Source: CAD feature listing. Evaluate the final solid. Frame: model axes, mm. Coordinates: 2 decimals unless noted, no trailing zeros. Order: outer loops, then holes, each group sorted by start corner. A loop starts at its lowest first (then second) coordinate and runs counter-clockwise, first axis right, second up.
```python
from build123d import *

# Parameters (mm, degrees)
SKETCH1_W           = 20
SKETCH1_H           = 20
BOSS_EXTRUDE1_DEPTH = 116
SKETCH1_5_R         = 1
CUT_EXTRUDE1_DEPTH  = 10
SKETCH4_R           = 1
CUT_EXTRUDE2_DEPTH  = 10
SKETCH5_R           = 2.5
CUT_EXTRUDE3_DEPTH  = 21
SKETCH6_R           = 5
CUT_EXTRUDE4_DEPTH  = 10


with BuildPart() as part:
    # Sketch1 → Boss-Extrude1 (new body)
    with BuildSketch(Plane.XY):
        with Locations((10, 10)):
            Rectangle(SKETCH1_W, SKETCH1_H)
    extrude(amount=BOSS_EXTRUDE1_DEPTH)

    # Sketch1_5 → Cut-Extrude1 (cut)
    with BuildSketch(Plane.XY):
        with Locations((15, 10)):
            Circle(SKETCH1_5_R)
        with Locations((5, 10)):
            Circle(SKETCH1_5_R)
    extrude(amount=CUT_EXTRUDE1_DEPTH, mode=Mode.SUBTRACT)

    # Sketch4 → Cut-Extrude2 (cut)
    with BuildSketch(Plane.XY.offset(116)):
        with Locations((5, 10)):
            Circle(SKETCH4_R)
        with Locations((15, 10)):
            Circle(SKETCH4_R)
    extrude(amount=-CUT_EXTRUDE2_DEPTH, mode=Mode.SUBTRACT)

    # Sketch5 → Cut-Extrude3 (cut, through all)
    with BuildSketch(Plane(origin=(20, 0, 0), x_dir=(0, 0, -1), z_dir=(1, 0, 0))):
        with Locations((-98, 10)):
            Circle(SKETCH5_R)
        with Locations((-18, 10)):
            Circle(SKETCH5_R)
    extrude(amount=-CUT_EXTRUDE3_DEPTH, mode=Mode.SUBTRACT)

    # Sketch6 → Cut-Extrude4 (cut)
    with BuildSketch(Plane(origin=(20, 0, 0), x_dir=(0, 0, -1), z_dir=(1, 0, 0))):
        with Locations((-98, 10)):
            Circle(SKETCH6_R)
        with Locations((-18, 10)):
            Circle(SKETCH6_R)
    extrude(amount=-CUT_EXTRUDE4_DEPTH, mode=Mode.SUBTRACT)


solid = part.part
```
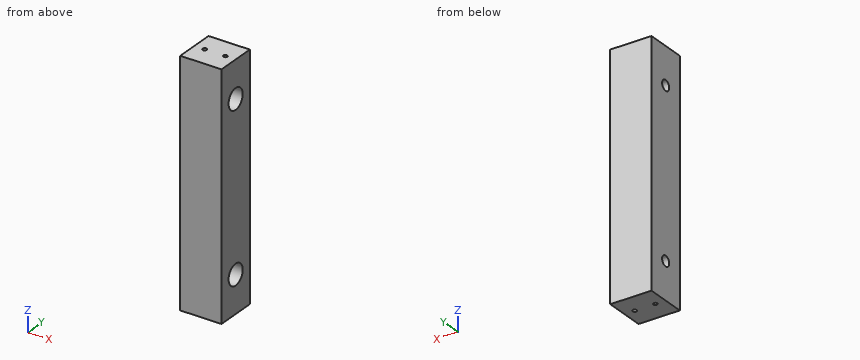
Q1. Pin query (flat end, axial travel): P1, Ø5, axis at y = 11, z = 16, coming from the +X side; P2, Ø1.8, axis at x = 15, y = 10, coming from the +Z side; P3, Ø12, axis at x = 12, y = 12.5, coming from the -Z side; P4, Ø1.6, axis at x = 5, y = 10, coming from the -Z side. Return the tip coordinate at first contact, or that it passes through.
Solutions:
P1: stops at x = 10
P2: stops at z = 106
P3: stops at z = 0
P4: stops at z = 10
Q2. Section query D-D on x = 5. Output: boundary loops of the cut face in (y, z).
Solutions:
outline: (0, 0) - (9, 0) - (9, 10) - (11, 10) - (11, 0) - (20, 0) - (20, 116) - (11, 116) - (11, 106) - (9, 106) - (9, 116) - (0, 116) - close; hole circle Ø5 at (10, 18); hole circle Ø5 at (10, 98)
Q3. Section query C-C on y = 10. Give the number of separate pieces and of enclosed holes in the cut face, plus the area to 3 significant figures.
Solutions:
separate pieces: 3
enclosed holes: 0
area: 1,940 mm2
Q4. Section query B-B on x = 15. Output: boundary loops of the cut face in (y, z).
Solutions:
outline: (0, 0) - (9, 0) - (9, 10) - (11, 10) - (11, 0) - (20, 0) - (20, 116) - (11, 116) - (11, 106) - (9, 106) - (9, 116) - (0, 116) - close; hole circle Ø10 at (10, 18); hole circle Ø10 at (10, 98)
Q5. Section query A-A on z = 18. Output: boundary loops of the cut face in (x, y).
Solutions:
outline: (0, 0) - (20, 0) - (20, 5) - (10, 5) - (10, 7.5) - (0, 7.5) - close; (0, 12.5) - (10, 12.5) - (10, 15) - (20, 15) - (20, 20) - (0, 20) - close
Q6. Material intervals for line 1 along Y through (x, z) = (15, 114); line 2 along Z through (x, y) = (18.25, 13.75); line 3 along Y through (x, z) = (13.25, 98), sorted ascending.
Solutions:
line 1: y = 0 to 9, 11 to 20
line 2: z = 0 to 14.69, 21.31 to 94.69, 101.31 to 116
line 3: y = 0 to 5, 15 to 20
